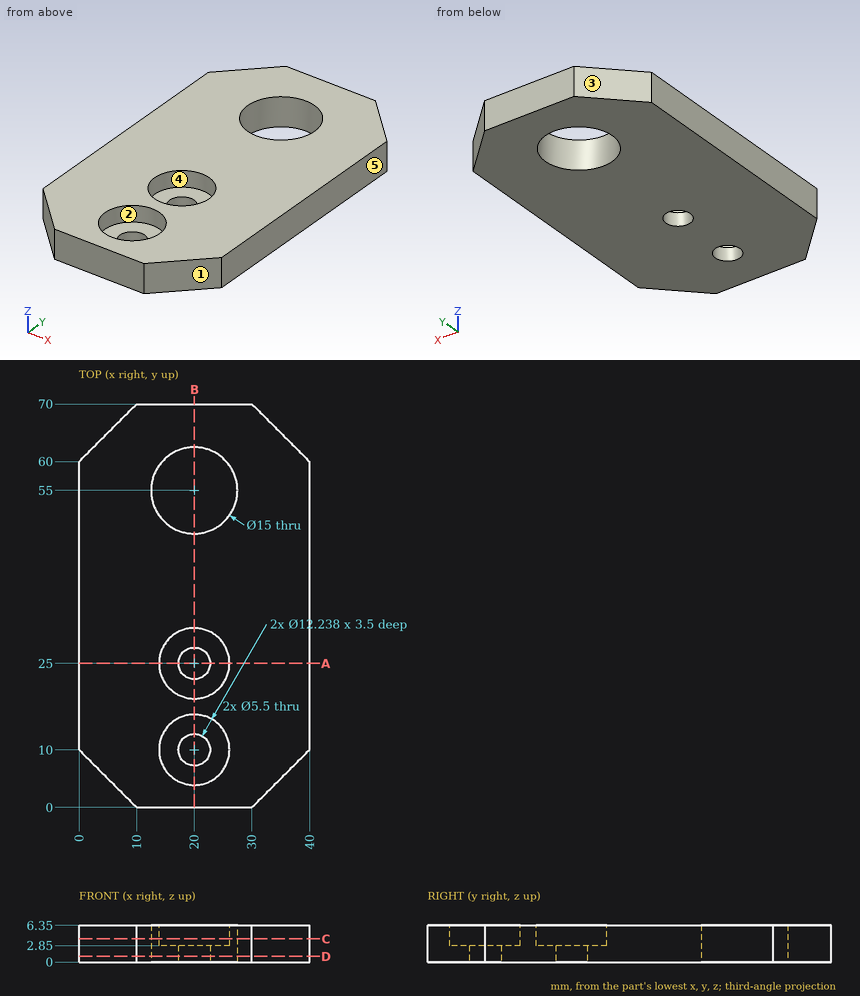
The figure shows three views and two pictorial views of one solid part (mm, origin at its lowest corner). Answer the questions. A direction names the side the tool comes from. Round coordinates to 2 decimals unless told otherwise and drop trailing zeros. Write each loop counter-clockwise with the first axis right and the second up, starting at its lowest first coordinate (ties: lowest second). Pieces come first, ordered by that corner, then holes. Notation, with made-up numbers: (-11.75, -39) - (45.25, -39) arc R22 ccw to (45.25, -23) - close; hole circle Ø7 at (28, 32). An arc over 180 degrees is marked (long way). Use one line per item in the form item = value. Start each with the question number.
Item 1: A cutting plane is placed at D-D (z = 1). Write down the section's boundary in (x, y), plus the area to 3 significant figures.
Item 2: A tool of negligible diameter and unlimited length cuts with its end or side. For the marked faces 4 and 5, from which of +Z, -Z, +X, -X, +Y, -Y can it reach the whole face along a straight path? Write none if from no direction.
Item 3: A cutting plane is placed at A-A (y = 25). Write down the section's boundary in (x, z).
Item 4: A flat-ended cylindrical pin translates along its axis: pin 1 Ø6.5 at (x, y) = (20, 10) entering from +Z. Find the tip coordinate at first contact, or state that the pin passes through.
Item 5: Find the intervals of material crossed by line 1 (Y direction, x = 20, z = 4.9); line 2 (Y direction, x = 20, z = 0.9); line 3 (X direction, y = 51.5, z = 2.75), in increasing order. Write a range as [from, to].
Item 6: Determine the mould class of the marked faces 1, 2 and 3 for opening direction X: +X half, -X half, draft (parallel to the pull), parting line (faces both ways), or undercut.
Item 7: A cutting plane is placed at C-C (z = 4). Write down the section's boundary in (x, y), plus the area to 3 significant figures.
Item 8: A cutting plane is placed at B-B (x = 20). Write down the section's boundary in (y, z), plus the area to 3 significant figures.
The answers:
q1.outline = (0, 10) - (10, 0) - (30, 0) - (40, 10) - (40, 60) - (30, 70) - (10, 70) - (0, 60) - close; hole circle Ø15 at (20, 55); hole circle Ø5.5 at (20, 10); hole circle Ø5.5 at (20, 25)
q1.area = 2,380 mm^2
q2.face_4 = +Z
q2.face_5 = +Z, -Z, +X, +Y, -Y
q3.outline = (0, 0) - (17.25, 0) - (17.25, 2.85) - (13.88, 2.85) - (13.88, 6.35) - (0, 6.35) - close; (22.75, 0) - (40, 0) - (40, 6.35) - (26.12, 6.35) - (26.12, 2.85) - (22.75, 2.85) - close
q4.pin_1 = 2.85
q5.line_1 = [0, 3.88], [16.12, 18.88], [31.12, 47.5], [62.5, 70]
q5.line_2 = [0, 7.25], [12.75, 22.25], [27.75, 47.5], [62.5, 70]
q5.line_3 = [0, 13.37], [26.63, 40]
q6.face_1 = +X half
q6.face_2 = undercut
q6.face_3 = -X half
q7.outline = (0, 10) - (10, 0) - (30, 0) - (40, 10) - (40, 60) - (30, 70) - (10, 70) - (0, 60) - close; hole circle Ø15 at (20, 55); hole circle Ø12.24 at (20, 10); hole circle Ø12.24 at (20, 25)
q7.area = 2,190 mm^2
q8.outline = (0, 0) - (7.25, 0) - (7.25, 2.85) - (3.88, 2.85) - (3.88, 6.35) - (0, 6.35) - close; (12.75, 0) - (22.25, 0) - (22.25, 2.85) - (18.88, 2.85) - (18.88, 6.35) - (16.12, 6.35) - (16.12, 2.85) - (12.75, 2.85) - close; (27.75, 0) - (47.5, 0) - (47.5, 6.35) - (31.12, 6.35) - (31.12, 2.85) - (27.75, 2.85) - close; (62.5, 0) - (70, 0) - (70, 6.35) - (62.5, 6.35) - close
q8.area = 232 mm^2
